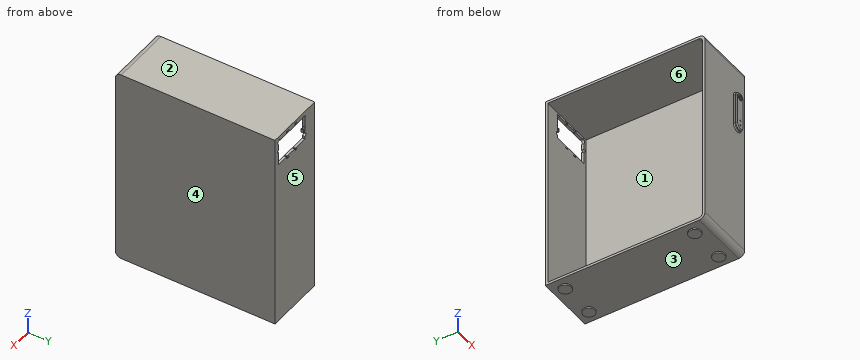
from build123d import *

# Parameters (mm, degrees)
F0_W      = 800
F0_H      = 1000
F1_DEPTH  = 300
F2_R      = 30
F4_DEPTH  = 287.5
F5_R      = 2.162666
F6_DEPTH  = 25
F8_DEPTH  = 15
F9_SIZE   = 5
F10_R     = 15
F11_DEPTH = 2
F12_R     = 3.75
F13_DEPTH = 20
F14_R     = 30
F15_DEPTH = 7.5


with BuildPart() as f1:
    # F0 (on Right) → F1 (new body)
    with BuildSketch(Plane.YZ):
        Rectangle(F0_W, F0_H)
    extrude(amount=F1_DEPTH)

    # F2
    f2_edges = [f1.edges().sort_by_distance(p)[0] for p in [
        (150, -400, 500),
        (150, -400, -500),
    ]]
    fillet(f2_edges, radius=F2_R)

    # F3 (on face) → F4 (cut)
    with BuildSketch(Plane(origin=(0, 0, 0), x_dir=(0, -1, 0), z_dir=(-1, 0, 0))):
        with BuildLine():
            Line((-387.5, 487.5), (-387.5, -487.5))
            Line((-387.5, -487.5), (367.5, -487.5))
            ThreePointArc((367.5, -487.5), (381.642136, -481.642136), (387.5, -467.5))
            Line((387.5, -467.5), (387.5, 467.5))
            ThreePointArc((387.5, 467.5), (381.642136, 481.642136), (367.5, 487.5))
            Line((367.5, 487.5), (-387.5, 487.5))
        make_face()
    extrude(amount=-F4_DEPTH, mode=Mode.SUBTRACT)

    # F5 (on face) → F6 (cut)
    with BuildSketch(Plane(origin=(0, 400, 0), x_dir=(-1, 0, 0), z_dir=(0, 1, 0))):
        with BuildLine():
            Line((-214.118924, 475), (-261.462748, 475))
            ThreePointArc((-261.462748, 475), (-276.918235, 474.874673), (-274.336556, 459.635818))
            Line((-274.336556, 459.635818), (-274.336556, 428.506063))
            ThreePointArc((-274.336556, 428.506063), (-281.158562, 421.684057), (-274.336556, 414.86205))
            Line((-274.336556, 414.86205), (-274.336556, 350))
            Line((-274.336556, 350), (-214.118924, 350))
            ThreePointArc((-214.118924, 350), (-212.70471, 349.414214), (-212.118924, 348))
            Line((-212.118924, 348), (-212.118924, 340))
            ThreePointArc((-212.118924, 340), (-211.533137, 338.585786), (-210.118924, 338))
            Line((-210.118924, 338), (-196.118924, 338))
            ThreePointArc((-196.118924, 338), (-194.118924, 340), (-196.118924, 342))
            Line((-196.118924, 342), (-206.118924, 342))
            ThreePointArc((-206.118924, 342), (-207.533137, 342.585786), (-208.118924, 344))
            Line((-208.118924, 344), (-208.118924, 348))
            ThreePointArc((-208.118924, 348), (-207.533137, 349.414214), (-206.118924, 350))
            Line((-206.118924, 350), (-152.166363, 350))
            ThreePointArc((-152.166363, 350), (-150.752149, 349.414214), (-150.166363, 348))
            Line((-150.166363, 348), (-150.166363, 340))
            ThreePointArc((-150.166363, 340), (-149.580576, 338.585786), (-148.166363, 338))
            Line((-148.166363, 338), (-134.166363, 338))
            ThreePointArc((-134.166363, 338), (-132.166363, 340), (-134.166363, 342))
            Line((-134.166363, 342), (-144.166363, 342))
            ThreePointArc((-144.166363, 342), (-145.580576, 342.585786), (-146.166363, 344))
            Line((-146.166363, 344), (-146.166363, 348))
            ThreePointArc((-146.166363, 348), (-145.580576, 349.414214), (-144.166363, 350))
            Line((-144.166363, 350), (-74.336556, 350))
            Line((-74.336556, 350), (-74.336556, 364.400569))
            ThreePointArc((-74.336556, 364.400569), (-65.336556, 373.400569), (-74.336556, 382.400569))
            Line((-74.336556, 382.400569), (-74.336556, 388.44103))
            ThreePointArc((-74.336556, 388.44103), (-74.922342, 389.855244), (-76.336556, 390.44103))
            Line((-76.336556, 390.44103), (-84.336852, 390.44103))
            ThreePointArc((-84.336852, 390.44103), (-85.751066, 391.026817), (-86.336852, 392.44103))
            Line((-86.336852, 392.44103), (-86.336852, 406.44103))
            ThreePointArc((-86.336852, 406.44103), (-84.336704, 408.441178), (-82.336556, 406.44103))
            Line((-82.336556, 406.44103), (-82.336556, 396.44103))
            ThreePointArc((-82.336556, 396.44103), (-81.750769, 395.026817), (-80.336556, 394.44103))
            Line((-80.336556, 394.44103), (-76.336556, 394.44103))
            ThreePointArc((-76.336556, 394.44103), (-74.922342, 395.026817), (-74.336556, 396.44103))
            Line((-74.336556, 396.44103), (-74.336556, 413.516909))
            Line((-74.336556, 413.516909), (-71.336556, 413.516909))
            ThreePointArc((-71.336556, 413.516909), (-70.336556, 414.516909), (-71.336556, 415.516909))
            Line((-71.336556, 415.516909), (-74.336556, 415.516909))
            Line((-74.336556, 415.516909), (-74.336556, 473))
            Line((-74.336556, 473), (-71.336556, 473))
            ThreePointArc((-71.336556, 473), (-70.629449, 473.292893), (-70.336556, 474))
            ThreePointArc((-70.336556, 474), (-70.629449, 474.707107), (-71.336556, 475))
            Line((-71.336556, 475), (-74.336556, 475))
            Line((-74.336556, 475), (-81.430964, 475))
            ThreePointArc((-81.430964, 475), (-84.930964, 478.5), (-88.430964, 475))
            Line((-88.430964, 475), (-144.166363, 475))
            ThreePointArc((-144.166363, 475), (-145.580576, 475.585786), (-146.166363, 477))
            Line((-146.166363, 477), (-146.166363, 481))
            ThreePointArc((-146.166363, 481), (-145.580576, 482.414214), (-144.166363, 483))
            Line((-144.166363, 483), (-134.166363, 483))
            ThreePointArc((-134.166363, 483), (-132.166363, 485), (-134.166363, 487))
            Line((-134.166363, 487), (-148.166363, 487))
            ThreePointArc((-148.166363, 487), (-149.580576, 486.414214), (-150.166363, 485))
            Line((-150.166363, 485), (-150.166363, 477))
            ThreePointArc((-150.166363, 477), (-150.752149, 475.585786), (-152.166363, 475))
            Line((-152.166363, 475), (-206.118924, 475))
            ThreePointArc((-206.118924, 475), (-207.533137, 475.585786), (-208.118924, 477))
            Line((-208.118924, 477), (-208.118924, 481))
            ThreePointArc((-208.118924, 481), (-207.533137, 482.414214), (-206.118924, 483))
            Line((-206.118924, 483), (-196.118924, 483))
            ThreePointArc((-196.118924, 483), (-194.118924, 485), (-196.118924, 487))
            Line((-196.118924, 487), (-210.118924, 487))
            ThreePointArc((-210.118924, 487), (-211.533137, 486.414214), (-212.118924, 485))
            Line((-212.118924, 485), (-212.118924, 477))
            ThreePointArc((-212.118924, 477), (-212.70471, 475.585786), (-214.118924, 475))
        make_face()
        with Locations((-269.137114, 483.943254)):
            Circle(F5_R)
    extrude(amount=-F6_DEPTH, mode=Mode.SUBTRACT)

    # F7 (on face) → F8 (join)
    with BuildSketch(Plane.XZ.offset(400)):
        with BuildLine():
            ThreePointArc((244.205779, 341.809909), (226.528109, 334.487578), (219.205779, 316.809909))
            Line((219.205779, 316.809909), (219.205779, 166.809909))
            ThreePointArc((219.205779, 166.809909), (226.528109, 149.132239), (244.205779, 141.809909))
            ThreePointArc((244.205779, 141.809909), (261.883448, 149.132239), (269.205779, 166.809909))
            Line((269.205779, 166.809909), (269.205779, 316.809909))
            ThreePointArc((269.205779, 316.809909), (261.883448, 334.487578), (244.205779, 341.809909))
        make_face()
    extrude(amount=F8_DEPTH)

    # F9
    f9_edges = [f1.edges().sort_by_distance(p)[0] for p in [
        (219.205779, -407.5, 316.809909),
        (219.205779, -407.5, 166.809909),
        (219.205779, -400, 241.809909),
        (219.205779, -415, 241.809909),
    ]]
    chamfer(f9_edges, length=F9_SIZE)

    # F10 (on face) → F11 (join)
    with BuildSketch(Plane.XZ.offset(415)):
        with Locations((244.205779, 316.809909)):
            Circle(F10_R)
        with BuildLine():
            ThreePointArc((236.002863, 323.692972), (237.958707, 323.864086), (238.129821, 321.908243))
            ThreePointArc((238.129821, 321.908243), (244.205779, 308.878309), (250.281737, 321.908243))
            ThreePointArc((250.281737, 321.908243), (250.452851, 323.864086), (252.408694, 323.692972))
            ThreePointArc((252.408694, 323.692972), (244.205779, 306.101763), (236.002863, 323.692972))
        make_face(mode=Mode.SUBTRACT)
        with BuildLine():
            ThreePointArc((244.899914, 316.809909), (244.205779, 316.115774), (243.511644, 316.809909))
            Line((243.511644, 316.809909), (243.511644, 327.513516))
            ThreePointArc((243.511644, 327.513516), (244.205779, 328.207651), (244.899914, 327.513516))
            Line((244.899914, 327.513516), (244.899914, 316.809909))
        make_face(mode=Mode.SUBTRACT)
    extrude(amount=F11_DEPTH)

    # F12 (on face) → F13 (cut)
    with BuildSketch(Plane.XZ.offset(415)):
        with Locations((244.205779, 191.809909)):
            Circle(F12_R)
        with Locations((244.205779, 166.809909)):
            Circle(F12_R)
    extrude(amount=-F13_DEPTH, mode=Mode.SUBTRACT)

    # F14 (on face) → F15 (join)
    with BuildSketch(Plane(origin=(0, 0, -500), x_dir=(1, 0, 0), z_dir=(0, 0, -1))):
        with Locations((240, -340)):
            Circle(F14_R)
        with Locations((60, -340)):
            Circle(F14_R)
        with Locations((240, 310)):
            Circle(F14_R)
        with Locations((58.350662, 310)):
            Circle(F14_R)
    extrude(amount=F15_DEPTH)


solid = f1.part
Model file for the job. Use its own axes, mm. Face numbers are marked on the shaded views. A direction names the side the tool comes from. Round coordinates to 2 decimals unless told otherwise and drop trailing zeros. Order: outer loops, then holes, each group sorted by start corner. A loop starts at its lowest first (then second) coordinate and runs counter-clockwise, first axis right, second up. Notation, with made-up numbers: M 52,69.5 L 61,69.5 A32 ccw 61,100.5 Z; hole C 69,67.5 d10. An arc over 180 degrees is marked long. Write each question's results on one line, items separated by ' | '. Start each with the question number.
(1) Saw through at B-B, the plane z = -278. Give the cut face in (x, y).
(2) Probe probe 1 along Z at (x, y) = (223, -284); probe 2 along Y at (x, z) = (107, 195); probe 3 along Y at (x, z) = (263.5, 438.5). List the from-to ranges inside material, lowest first. Write a range as from..to.
(3) Saw through at A-A, the plane y = 273.5. Give the cut face in (x, z).
(4) Which spindle directions (+Z, -Z, +X, -X, +Y, -Y) get a long thin tool onto all of the face, cutting with end or side? Do the marked faces 1, 2 and 3. Say none if no direction does.
(5) Saw through at C-C, the plane z = 285.5. Give the cut face in (x, y), then the cut area to 3 significant figures.
(6) Drop flat-ended pins along their axis: pin 1 (5.5 mm diameter, centred on y = -408.5, z = 265, fed in from +X); pin 2 (3.5 mm diameter, centred on x = 73, y = 390.5, fed in from -Z); pin 3 (2 mm diameter, centred on y = 280.5, z = -257, fed in from -X); pin 4 (3 mm diameter, centred on y = 396, z = 401, fed in from -X). Give the stop position or say it passes through.
(7) Two-plate mould, pull along Y, no slides. Class the marked faces 4, 5 and 6: pulls with the +Y half, pulls with the -Y half, needs draft (parallel to the pull), parting line crosses it, or undercut.
Established:
1) outline: M 0,-400 L 300,-400 L 300,400 L 0,400 L 0,387.5 L 287.5,387.5 L 287.5,-387.5 L 0,-387.5 Z
2) probe 1: z = -500..-487.5, 487.5..500 | probe 2: y = -400..-387.5, 387.5..400 | probe 3: y = -400..-387.5
3) outline: M 0,-500 L 300,-500 L 300,500 L 0,500 L 0,487.5 L 287.5,487.5 L 287.5,-487.5 L 0,-487.5 Z
4) face 1: -X | face 2: +Z, +X, -X, +Y, -Y | face 3: -Z
5) outline: M 0,-400 L 214.21,-400 L 219.21,-405 L 219.21,-410 L 224.21,-415 L 264.21,-415 L 269.21,-410 L 269.21,-405 L 274.21,-400 L 300,-400 L 300,400 L 0,400 L 0,387.5 L 287.5,387.5 L 287.5,-387.5 L 0,-387.5 Z | area: 17,900 mm^2
6) pin 1: stops at x = 269.21 | pin 2: stops at z = -500 | pin 3: stops at x = 287.5 | pin 4: stops at x = 0
7) face 4: needs draft | face 5: pulls with the +Y half | face 6: undercut
